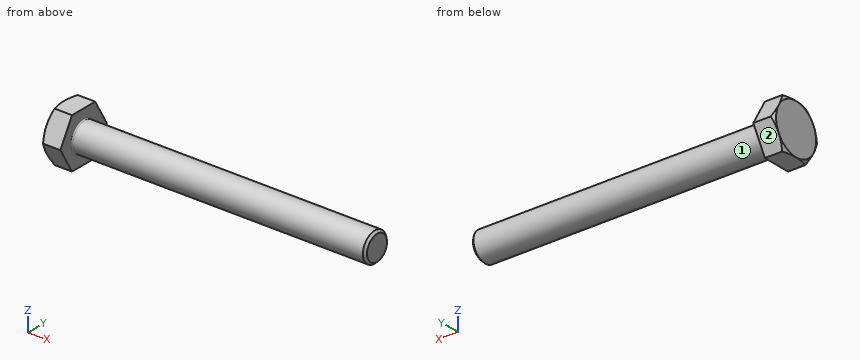
Autodesk Inventor part; units mm, degrees
ref_plane "Work Plane1" through (1.525, 0, 0) normal (0, 0, 1) x (1, 0, 0)
ref_plane "YZ Plane" through (0, 0, 0) normal (1, 0, 0) x (0, 1, 0)
ref_plane "XZ Plane" through (0, 0, 0) normal (0, 1, 0) x (-1, 0, 0)
sketch "Sketch1" plane through (0, 0, 0) normal (0, 0, 1) x (1, 0, 0)
  line L0 (0, 10) -> (200, 10)
  line L1 (200, 10) -> (200, 0)
  line L2 (200, 0) -> (0, 0)
  line L3 (-40, 0) -> (240, 0)
  line L4 (0, -2) -> (0, 12)
  line L5 (0, 10) -> (0, 0)
  dimension "d2" = 20
  dimension "d59" = 200
revolve "Body" add sketch "Sketch1" angle 360 about axis through (200, 0, 0) along (-1, 0, 0)
sketch "Sketch2" plane through (0, 0, 0) normal (-1, 0, 0) x (0, 0, 1)
  line L0 (0, 19.6299) -> (17, 9.815)
  line L1 (17, 9.815) -> (17, -9.815)
  line L2 (17, -9.815) -> (0, -19.6299)
  line L3 (0, -19.6299) -> (-17, -9.815)
  line L4 (-17, -9.815) -> (-17, 9.815)
  line L5 (-17, 9.815) -> (0, 19.6299)
  line L6 (-23.8, 0) -> (23.8, 0)
  line L7 (0, 27.4819) -> (0, -27.4819)
  point P0 (0, 0)
  point P1 (0, 0)
  dimension "d11" = 34
extrude "Head" add sketch "Sketch2" along normal blind 13.4
sketch "Sketch4" plane through (0, 0, 0) normal (0, 0, 1) x (1, 0, 0)
  line L0 (-11.437, 20.4) -> (-13.4, 17)
  line L1 (-1.1, 0) -> (-0.234, 0)
  line L2 (-16.0332, 0) -> (2.3992, 0)
  line L3 (-13.4, 20.4) -> (-11.437, 20.4)
  line L4 (-13.4, 17) -> (-13.4, 20.4)
  line L5 (0, 24.48) -> (0, -4.08)
  dimension "d65" = 34
  dimension "d67" = 30
  dimension "d68" = 40.8
  dimension "d69" = 13.4
revolve "Chamfer1" cut sketch "Sketch4" angle 360 about axis through (-1.1, 0, 0) along (1, 0, 0)
thread "Thread"
chamfer "Chamfer2" distance 1.5336 distance2 1.5337 1 edges at (200, -10, 0) measured on face at (200, 1.182, 2.3698)
fillet "Fillet" radius 0.8 1 edges at (0, -10, 0)
ref_plane "Work Plane1" through (1.525, 0, 0) normal (0, 0, 1) x (1, 0, 0)
equation "\"d2\" = GD"
equation "\"d59\" = NLG"
equation "\"d11\" = SW"
equation "\"d3\" = KOH"
equation "\"d15\" = GEL"
equation "\"d6\" = -0.5 * SPD + 0.5 * GD"
equation "\"d71\" = RR1"
equation "\"d65\" = SW"
equation "\"d67\" = ANG1"
equation "\"d68\" = 1.2 * SW"
equation "\"d69\" = KOH"
equation "\"NLG\" = 200"
equation "\"GD\" = NND"
equation "\"KOH\" = 13.4"
equation "\"GEL\" = 52"
equation "\"SW\" = 34"
equation "\"SW0\" = SW"
equation "\"SPD\" = NND - 1.2269 * PTC"
equation "\"SD\" = 0"
equation "\"ANG1\" = 30deg"
equation "\"GAL\" = 0.61345 * PTC"
equation "\"GUL\" = 0.61345 * PTC"
equation "\"RR\" = 0.1"
equation "\"RR1\" = 0.8"
equation "\"GD1\" = THREADDIA - 1.2269 * PTC"
equation "\"TOA\" = 30deg"
equation "\"PTC\" = 2.5"
equation "\"KOH1\" = 8.8"
equation "\"E0\" = 1.155 * SW"
properties part number "ANSI B18.2.3.6M - M20 x 2.5 x 200" material "Steel, Mild"
Geometry check sheet. Reference: the model listing, model coordinates, mm. Face numbers are marked on the shaded views. A direction names the side the tool comes from. Round coordinates to 2 decimals unless told otherwise and drop trailing zeros. Loops run counter-clockwise (first coordinate to the right, second up) from the corner with the lowest first, then second, coordinate; pieces in that order, holes last. Notation, with made-up numbers: (-27.75, 77) - (-12.75, 77) arc R15 ccw to (-12.75, 84) - close; hole circle Ø11 at (-15.75, 7.5). An arc over 180 degrees is marked (long way). Write each question's results on one line, items separated by ' | '. Start each with the question number.
Q1. Gauge pin test, flat ends, axial feed: P1, Ø3, axis at x = 112.5, z = -3.5, coming from the -Y side; P2, Ø10, axis at y = -8.5, z = -0.5, coming from the +X side; P3, Ø3, axis at x = 166, z = -3, coming from the -Y side; P4, Ø10, axis at x = 164.5, y = 8, coming from the -Z side. Record the tip position at first contact, or that the pin passes through.
Q2. Thickness scan on line 1 (Y direction, x = 11.5, z = 2); line 2 (Y direction, x = 33.5, z = 0.5). Record the ranges inside material, lowest first. Write a range as [from, to].
Q3. Cross-section at A-A on x = 112.5. Enter the section's corners in (y, z), and give its area (3 significant figures).
Q4. Access from +Z, -Z, +X, -X, +Y, -Y to the whole of each face (thin tool, end or side, straight path). Record for the marked faces 1 and 2.
Answers below:
1) P1: stops at y = -9.8 | P2: stops at x = 200 | P3: stops at y = -9.89 | P4: stops at z = -9.54
2) line 1: y = [-9.8, 9.8] | line 2: y = [-9.99, 9.99]
3) outline: circle Ø20 at (0, 0) | area: 314 mm²
4) face 1: +X | face 2: -Z, +X, -X, +Y
